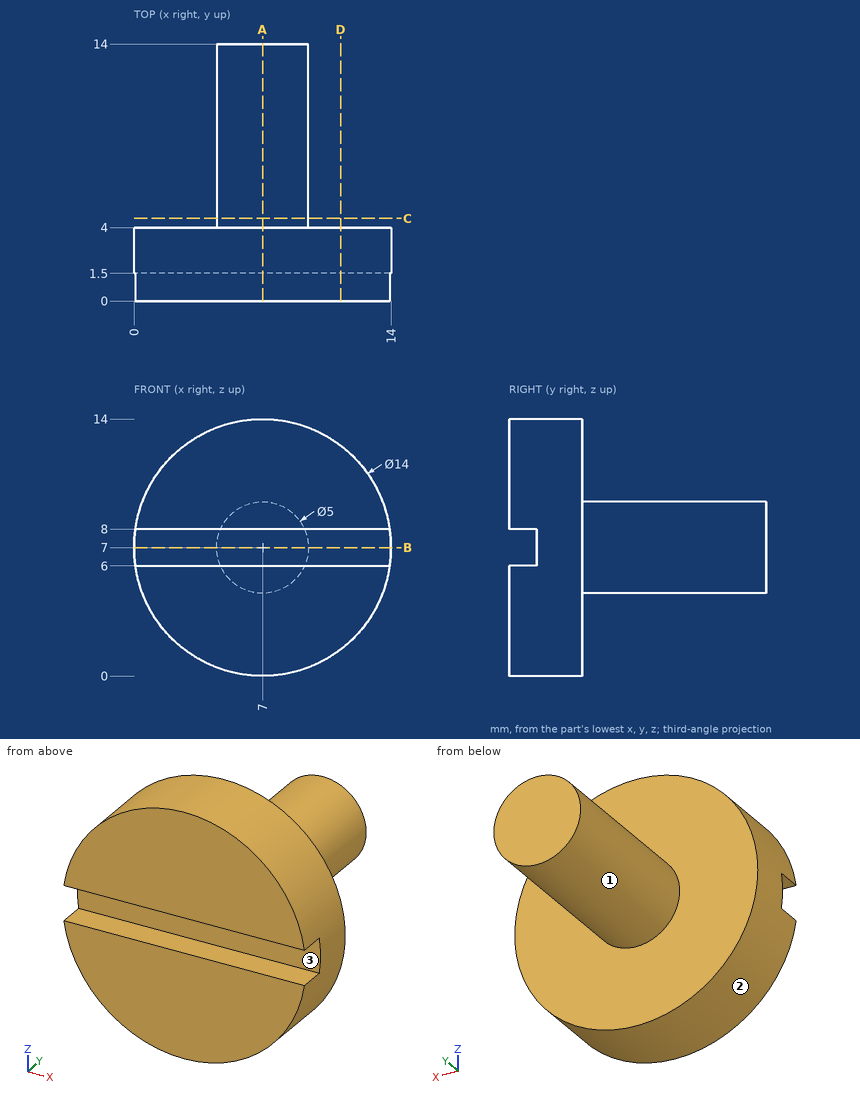
Design review of the part shown in the three views and the two pictorial views. Dimensions are in mm from the part's minimum x, y and z. A direction names the side the tool comes from. Round coordinates to 2 decimals unless told otherwise and drop trailing zeros. Loops run counter-clockwise (first coordinate to the right, second up) from the corner with the lowest first, then second, coordinate; pieces in that order, holes last. Notation, with made-up numbers: (50.5, 21.5) - (91.5, 21.5) arc R26 ccw to (91.5, 58.5) - close; hole circle Ø6 at (26.5, 69). An arc over 180 degrees is marked (long way). Use CSV: the item, a comma, the result in double quotes.
(1) Take a section at A-A, the plane x = 7. Give the boundary of the cut face in (y, z).
Working result:
outline,"(0, 0) - (4, 0) - (4, 4.5) - (14, 4.5) - (14, 9.5) - (4, 9.5) - (4, 14) - (0, 14) - (0, 8) - (1.5, 8) - (1.5, 6) - (0, 6) - close"
(2) Take a section at C-C, the plane y = 4.5. Give the boundary of the cut face in (x, z).
Working result:
outline,"circle Ø5 at (7, 7)"
(3) Take a section at D-D, the plane x = 11.25. Give the boundary of the cut face in (y, z), plus the area to 3 significant figures.
Working result:
outline,"(0, 1.44) - (4, 1.44) - (4, 12.56) - (0, 12.56) - (0, 8) - (1.5, 8) - (1.5, 6) - (0, 6) - close"
area,"41.5 mm^2"
(4) Machinability: for the marked faces 1, 2 and 3, which of the approach directions +Z, -Z, +X, -X, +Y, -Y give a long, thin tool a straight path to every point of the face, cutting with its end or side? Answer none if there is none.
Working result:
face 1,"+Y"
face 2,"+Y, -Y"
face 3,"+X, -X, -Y"
(5) For line 1 (Y direction, x = 10.75, z = 12.75); line 2 (Z direction, x = 11, y = 1); line 3 (X direction, y = 4.25, z = 8), list the stretches that pass through material, from the lowest coordinate up.
Working result:
line 1,"y = 0 to 4"
line 2,"z = 1.26 to 6, 8 to 12.74"
line 3,"x = 4.71 to 9.29"
(6) Clearance check with flat-ended pins moving along their axes: P1, Ø0.6, axis at x = 4, z = 7.5, coming from the -Y side; P2, Ø1.6, axis at x = 4.5, y = 1, coming from the -Z side; P3, Ø4, axis at x = 9, y = 8.5, coming from the -Z side. State where each tip first meets the part, or that it passes through.
Working result:
P1,"stops at y = 1.5"
P2,"stops at z = 0.21"
P3,"stops at z = 4.5"
(7) Take a section at B-B, the plane z = 7. Give the boundary of the cut face in (x, y).
Working result:
outline,"(0, 1.5) - (14, 1.5) - (14, 4) - (9.5, 4) - (9.5, 14) - (4.5, 14) - (4.5, 4) - (0, 4) - close"
